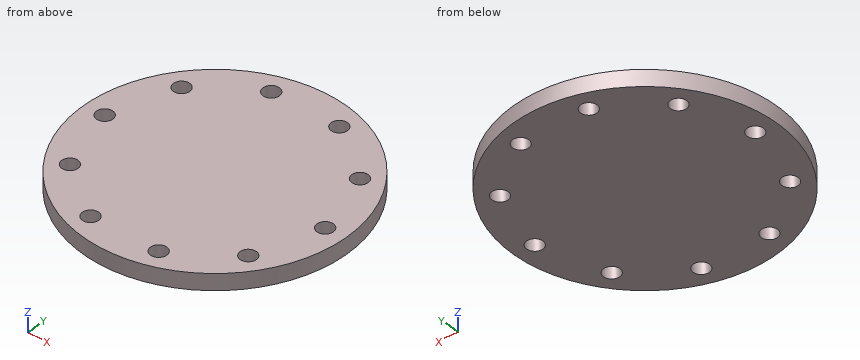
Autodesk Inventor part; units mm, degrees
ref_plane "YZ Plane" through (0, 0, 0) normal (1, 0, 0) x (0, 1, 0)
ref_plane "XZ Plane" through (0, 0, 0) normal (0, 1, 0) x (-1, 0, 0)
ref_plane "XY Plane" through (0, 0, 0) normal (0, 0, 1) x (1, 0, 0)
ref_plane "Work Plane1" through (0, 0, 0) normal (0, 0, 1) x (1, 0, 0)
sketch "Sketch1" plane through (0, 0, 0) normal (0, 0, 1) x (1, 0, 0)
  circle A0 centre (0, 0) radius 25.6348
  circle A1 centre (-6.7, 20.6205) radius 1.5875
  circle A2 centre (6.7, 20.6205) radius 1.5875
  circle A3 centre (17.5408, 12.7442) radius 1.5875
  circle A4 centre (21.6817, 0) radius 1.5875
  circle A5 centre (17.5408, -12.7442) radius 1.5875
  circle A6 centre (6.7, -20.6205) radius 1.5875
  circle A7 centre (-6.7, -20.6205) radius 1.5875
  circle A8 centre (-17.5408, -12.7442) radius 1.5875
  circle A9 centre (-21.6817, 0) radius 1.5875
  circle A10 centre (-17.5408, 12.7442) radius 1.5875
  point P0 (0, 0)
extrude "Extrusion1" add sketch "Sketch1" along normal blind 3.175
properties part number "topPlate" material "Polycarbonate, Clear"
Source: CAD feature listing. Evaluate the final solid. Frame: model axes, mm. Round coordinates to 2 decimals unless told otherwise and drop trailing zeros. Write each loop counter-clockwise with the first axis right and the second up, starting at its lowest first coordinate (ties: lowest second). Pieces come first, ordered by that corner, then holes. Notation, with made-up numbers: (28.5, 41.5) - (70.5, 41.5) arc R20 cw to (70.5, 61.5) - close; hole circle Ø6 at (48, 66). An arc over 180 degrees is marked (long way). Use CSV: the item, a comma, the result in double quotes. Start each with the question number.
(1) Cut plane A-A, the plane z = 2.25. Give the number of separate pieces and of enclosed holes in the cut face, and give its area (3 significant figures).
(2) Cut plane D-D, the plane y = 15.5. Return loops of the section in (x, z) (3 decimals).
(3) Material intervals for probe 1 along Y at (x, z) = (-7.5, 2.9); probe 2 along X at (y, z) = (-20, 0.3); probe 3 along Y at (x, z) = (17.5, 2.6), sorted ascending. Write a range as [from, to].
(4) First-contact query: pin 1 Ø1 at (y, z) = (-10.5, 2.5) entering from -X; pin 2 Ø1 at (y, z) = (-3.5, 1.5) entering from -X. Flat tips, straight axial feed; report the tip coordinate or a pass-through.
(5) Cut plane B-B, the plane y = -20. Return loops of the section in (x, z) (3 decimals), and give its area (3 significant figures).
(6) Cut plane C-C, the plane x = -6.7. Return loops of the section in (y, z) (3 decimals).
Geometry says:
1,separate pieces,"1"
1,enclosed holes,"10"
1,area,"1,990 mm²"
2,outline,"(-20.418, 0) - (20.418, 0) - (20.418, 3.175) - (-20.418, 3.175) - close"
3,probe 1,"[-24.51, -21.99], [-19.25, 19.25], [21.99, 24.51]"
3,probe 2,"[-16.04, -8.16], [-5.24, 5.24], [8.16, 16.04]"
3,probe 3,"[-18.73, -14.33], [-11.16, 11.16], [14.33, 18.73]"
4,pin 1,"x = -23.6"
4,pin 2,"x = -25.46"
5,outline,"(-16.036, 0) - (-8.161, 0) - (-8.161, 3.175) - (-16.036, 3.175) - close; (-5.239, 0) - (5.239, 0) - (5.239, 3.175) - (-5.239, 3.175) - close; (8.161, 0) - (16.036, 0) - (16.036, 3.175) - (8.161, 3.175) - close"
5,area,"83.3 mm²"
6,outline,"(-24.744, 0) - (-22.208, 0) - (-22.208, 3.175) - (-24.744, 3.175) - close; (-19.033, 0) - (19.033, 0) - (19.033, 3.175) - (-19.033, 3.175) - close; (22.208, 0) - (24.744, 0) - (24.744, 3.175) - (22.208, 3.175) - close"
